Input: part model. Units: mm. Frame: model coordinates. Face numbers are marked on the shaded views. A direction names the side the tool comes from. Coordinates: 2 decimals unless noted, no trailing zeros. Write each loop counter-clockwise with the first axis right and the second up, starting at its lowest first coordinate (ties: lowest second). Pieces come first, ordered by that corner, then holes. Notation, with made-up numbers: (71, 79) - (128, 79) arc R10 cw to (128, 89) - close; hole circle Ø7 at (76.5, 29). An arc over 180 degrees is marked (long way). Put each result on its own line as item: value. Start each with the question number.
1. Cut plane A-A, the plane x = -30. Return loops of the section in (y, z), and give its area (3 significant figures).
2. Cut plane B-B, the plane z = -6. Return loops of the section in (x, y).
3. Pin query (flat end, axial travel): pin 1 (4 mm diameter, centred on x = 2, y = 1.5, fed in from +Z); pin 2 (12 mm diameter, centred on x = 5.5, y = -39.5, fed in from -Z); pin 3 (6 mm diameter, centred on x = 11, y = 43.5, fed in from -Z). Return the tip coordinate at first contact, or that it passes through.
4. Access query for the marked faces 1, 2, 3 and 4. Directions: +Z, -Z, +X, -X, +Y, -Y. A direction counts if a zero-diameter tool reaches every point of the face in a straight line with its end or side. Return the directions, or none.
5. Cut plane C-C, the plane y = -16. Return loops of the section in (x, z), and give its area (3 significant figures).
6. Cut plane D-D, the plane z = -29. Return loops of the section in (x, y), and give its area (3 significant figures).
7. Line query: line 1 (Y direction, x = 10, z = -3); line 2 (Y direction, x = 10, z = 18); line 3 (Y direction, x = 10, z = -8). Output: solid intervals per line, ascending.
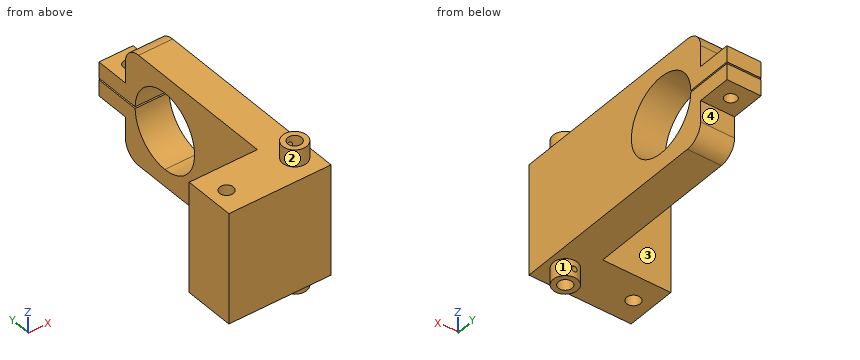
from build123d import *

# Parameters (mm, degrees)
CROQUIS1_R                                     = 22.5
SALIENTE_EXTRUIR1_DEPTH                        = 20
CROQUIS2_W                                     = 65
CROQUIS2_H                                     = 30
SALIENTE_EXTRUIR2_DEPTH                        = 40
CROQUIS4_W                                     = 1
CROQUIS4_H                                     = 60
CORTAR_EXTRUIR1_DEPTH                          = 40
TALADRO_DE_MARGEN_PARA_M61_D                   = 7
CROQUIS6_R                                     = 4
CORTAR_EXTRUIR2_DEPTH                          = 126.797456254
SALIENTE_EXTRUIR3_DEPTH                        = 10
SALIENTE_EXTRUIR3_DEPTH_BACK                   = 75
CROQUIS7_R                                     = 7.032700754
CROQUIS7_R_2                                   = 4.032700754
PERFORADOR_PARA_ROSCAR_PARA_MACHO_DE_ROS_D     = 3.3
PERFORADOR_PARA_ROSCAR_PARA_MACHO_DE_ROS_DEPTH = 5
PERFORADOR_PARA_ROSCAR_PARA_MACHO_DE_ROS_TIP   = 0.991420021
PERFORADOR_PARA_ROSCAR_PARA_MACHO_DE_2_D       = 3.3
PERFORADOR_PARA_ROSCAR_PARA_MACHO_DE_2_DEPTH   = 5
PERFORADOR_PARA_ROSCAR_PARA_MACHO_DE_2_TIP     = 0.991420021


with BuildPart() as part:
    # Croquis1 → Saliente-Extruir1 (new body)
    with BuildSketch(Plane(origin=(0, 0, 0), x_dir=(0, 0, -1), z_dir=(1, 0, 0))):
        with BuildLine():
            Line((-32.5, 0), (-32.5, -100))
            Line((-32.5, -100), (32.5, -100))
            Line((32.5, -100), (32.5, 0))
            Line((32.5, 0), (32.5, 19.863502686))
            ThreePointArc((32.5, 19.863502686), (29.571067812, 26.934570498), (22.5, 29.863502686))
            Line((22.5, 29.863502686), (10, 29.863502686))
            Line((10, 29.863502686), (10, 49.863502686))
            Line((10, 49.863502686), (-10, 49.863502686))
            Line((-10, 49.863502686), (-10, 29.863502686))
            Line((-10, 29.863502686), (-22.5, 29.863502686))
            ThreePointArc((-22.5, 29.863502686), (-29.571067812, 26.934570498), (-32.5, 19.863502686))
            Line((-32.5, 19.863502686), (-32.5, 0))
        make_face()
        Circle(CROQUIS1_R, mode=Mode.SUBTRACT)
    extrude(amount=SALIENTE_EXTRUIR1_DEPTH)

    # Croquis2 → Saliente-Extruir2 (add)
    with BuildSketch(Plane.ZY):
        with Locations((0, -85)):
            Rectangle(CROQUIS2_W, CROQUIS2_H)
    extrude(amount=SALIENTE_EXTRUIR2_DEPTH)

    # Croquis4 → Cortar-Extruir1 (cut)
    with BuildSketch(Plane.ZY):
        with Locations((0, 26.927828438)):
            Rectangle(CROQUIS4_W, CROQUIS4_H)
    extrude(amount=-CORTAR_EXTRUIR1_DEPTH, mode=Mode.SUBTRACT)

    # Taladro de margen para M61 (through all)
    with Locations(Plane(origin=(10, 39.863502686, -10), x_dir=(0, -1, 0), z_dir=(0, 0, -1))):
        with Locations((0, 0)):
            Hole(TALADRO_DE_MARGEN_PARA_M61_D / 2)

    # Croquis6 → Cortar-Extruir2 (cut, through all)
    with BuildSketch(Plane(origin=(0, 0, -32.5), x_dir=(-1, 0, 0), z_dir=(0, 0, -1))):
        with Locations((30, -85.367078143)):
            Circle(CROQUIS6_R)
        with Locations(Location((-10, -85.367078143, 0), (0, 0, 180))):
            Circle(CROQUIS6_R)
    extrude(amount=-CORTAR_EXTRUIR2_DEPTH, mode=Mode.SUBTRACT)

    # Croquis7 → Saliente-Extruir3 (add, two sides: drawn at the far end of the back side and taken through both)
    with BuildSketch(Plane.XY.offset(32.5).offset(-SALIENTE_EXTRUIR3_DEPTH_BACK)):
        with Locations((9.986743511, -85.396971367)):
            Circle(CROQUIS7_R)
        with Locations((9.986743511, -85.396971367)):
            Circle(CROQUIS7_R_2, mode=Mode.SUBTRACT)
    extrude(amount=SALIENTE_EXTRUIR3_DEPTH + SALIENTE_EXTRUIR3_DEPTH_BACK)

    # Perforador para roscar para macho de roscar para M4x0.71
    with Locations(Plane(origin=(9.940279275, -78.364424106, 37.5), x_dir=(0.999978174306, 0.006606883628, 0), z_dir=(-0.006606883628, 0.999978174306, 0))):
        with Locations((0, 0)):
            Hole(PERFORADOR_PARA_ROSCAR_PARA_MACHO_DE_ROS_D / 2, depth=PERFORADOR_PARA_ROSCAR_PARA_MACHO_DE_ROS_DEPTH)
            with Locations((0, 0, -(PERFORADOR_PARA_ROSCAR_PARA_MACHO_DE_ROS_DEPTH + PERFORADOR_PARA_ROSCAR_PARA_MACHO_DE_ROS_TIP / 2))):  # 118° drill point
                Cone(0, PERFORADOR_PARA_ROSCAR_PARA_MACHO_DE_ROS_D / 2, PERFORADOR_PARA_ROSCAR_PARA_MACHO_DE_ROS_TIP, mode=Mode.SUBTRACT)

    # Perforador para roscar para macho de 2
    with Locations(Plane(origin=(10.118803472, -78.365510632, -37.5), x_dir=(0.999823677927, -0.018777993951, 0), z_dir=(0.018777993951, 0.999823677927, 0))):
        with Locations((0, 0)):
            Hole(PERFORADOR_PARA_ROSCAR_PARA_MACHO_DE_2_D / 2, depth=PERFORADOR_PARA_ROSCAR_PARA_MACHO_DE_2_DEPTH)
            with Locations((0, 0, -(PERFORADOR_PARA_ROSCAR_PARA_MACHO_DE_2_DEPTH + PERFORADOR_PARA_ROSCAR_PARA_MACHO_DE_2_TIP / 2))):  # 118° drill point
                Cone(0, PERFORADOR_PARA_ROSCAR_PARA_MACHO_DE_2_D / 2, PERFORADOR_PARA_ROSCAR_PARA_MACHO_DE_2_TIP, mode=Mode.SUBTRACT)


solid = part.part
Report:
1. outline: (-100, -32.5) - (-89.37, -32.5) - (-89.37, 32.5) - (-100, 32.5) - close; (-81.37, -32.5) - (-70, -32.5) - (-70, 32.5) - (-81.37, 32.5) - close
1. area: 1,430 mm^2
2. outline: (-40, -100) - (20, -100) - (20, -21.69) - (0, -21.69) - (0, -70) - (-40, -70) - close; (0, 21.69) - (20, 21.69) - (20, 49.86) - (0, 49.86) - close; hole circle Ø8 at (-30, -85.37); hole circle Ø8 at (10, -85.37); hole circle Ø7 at (10, 39.86)
3. pin 1: stops at z = 32.5
3. pin 2: stops at z = -32.5
3. pin 3: stops at z = -10
4. face 1: -Z
4. face 2: +Z
4. face 3: +Z, -Z, -X, +Y
4. face 4: -Z, +X, -X, +Y
5. outline: (0, -32.5) - (20, -32.5) - (20, -15.82) - (0, -15.82) - close; (0, 15.82) - (20, 15.82) - (20, 32.5) - (0, 32.5) - close
5. area: 667 mm^2
6. outline: (-40, -100) - (20, -100) - (20, 27.46) - (0, 27.46) - (0, -70) - (-40, -70) - close; hole circle Ø8 at (-30, -85.37); hole circle Ø8 at (10, -85.37)
6. area: 3,650 mm^2
7. line 1: y = -100 to -89.37, -81.37 to -22.3, 22.3 to 36.36, 43.36 to 49.86
7. line 2: y = -100 to -89.37, -81.37 to -13.5, 13.5 to 29.86
7. line 3: y = -100 to -89.37, -81.37 to -21.03, 21.03 to 36.36, 43.36 to 49.86
